```python
from build123d import *

# Parameters (mm, degrees)
SKETCH1_W                       = 243.332
SKETCH1_H                       = 49.394999
BOSS_EXTRUDE1_DEPTH             = 1.905
SKETCH2_W                       = 8.466666667
SKETCH2_H                       = 8.466666667
SKETCH2_W_2                     = 8.466666666
BOSS_EXTRUDE2_DEPTH             = 9.525
CUT_EXTRUDE1_DEPTH              = 6.35
CHAMFER1_SIZE                   = 0.635
BOSS_EXTRUDE3_START             = -234.865333
BOSS_EXTRUDE3_DEPTH             = 234.865333
F_6_CLEARANCE_HOLE1_D           = 4.3053
F_6_CLEARANCE_HOLE1_CSINK_D     = 6.35
F_6_CLEARANCE_HOLE1_CSINK_ANGLE = 90


with BuildPart() as part:
    # Sketch1 → Boss-Extrude1 (new body)
    with BuildSketch(Plane.XY):
        with Locations((121.666, 24.6974995)):
            Rectangle(SKETCH1_W, SKETCH1_H)
    extrude(amount=BOSS_EXTRUDE1_DEPTH)

    # Sketch2 → Boss-Extrude2 (add)
    with BuildSketch(Plane.XY):
        with Locations((4.233333334, 45.161665666)):
            Rectangle(SKETCH2_W, SKETCH2_H)
        with Locations((127, 45.161665666)):
            Rectangle(SKETCH2_W_2, SKETCH2_H)
        with Locations((213.698666667, 45.161665666)):
            Rectangle(SKETCH2_W, SKETCH2_H)
    extrude(amount=-BOSS_EXTRUDE2_DEPTH)

    # Sketch3 → Cut-Extrude1 (cut)
    with BuildSketch(Plane(origin=(0, 49.394999, 0), x_dir=(1, 0, 0), z_dir=(0, 1, 0))):
        Polygon((1.058333333, 5.291666667), (4.233333333, 8.466666667), (7.408333333, 5.291666667), (4.233333333, 2.116666667), align=None)
        Polygon((123.825, 5.291666667), (127, 8.466666667), (130.175, 5.291666667), (127, 2.116666667), align=None)
        Polygon((210.523666667, 5.291666667), (213.698666667, 8.466666667), (216.873666667, 5.291666667), (213.698666667, 2.116666667), align=None)
    extrude(amount=-CUT_EXTRUDE1_DEPTH, mode=Mode.SUBTRACT)

    # Chamfer1
    chamfer1_edges = [part.edges().sort_by_distance(p)[0] for p in [
        (2.645833333, 43.044999, -3.704166667),
        (2.645833333, 43.044999, -6.879166667),
        (5.820833333, 43.044999, -6.879166667),
        (5.820833333, 43.044999, -3.704166667),
        (2.645833333, 49.394999, -3.704166667),
        (5.820833333, 49.394999, -3.704166667),
        (5.820833333, 49.394999, -6.879166667),
        (2.645833333, 49.394999, -6.879166667),
        (125.4125, 43.044999, -3.704166667),
        (125.4125, 43.044999, -6.879166667),
        (128.5875, 43.044999, -6.879166667),
        (128.5875, 43.044999, -3.704166667),
        (125.4125, 49.394999, -3.704166667),
        (128.5875, 49.394999, -3.704166667),
        (128.5875, 49.394999, -6.879166667),
        (125.4125, 49.394999, -6.879166667),
        (212.111166667, 43.044999, -3.704166667),
        (212.111166667, 43.044999, -6.879166667),
        (215.286166667, 43.044999, -6.879166667),
        (215.286166667, 43.044999, -3.704166667),
        (212.111166667, 49.394999, -3.704166667),
        (215.286166667, 49.394999, -3.704166667),
        (215.286166667, 49.394999, -6.879166667),
        (212.111166667, 49.394999, -6.879166667),
    ]]
    chamfer(chamfer1_edges, length=CHAMFER1_SIZE)


with BuildPart() as boss_extrude3_tool:
    # Sketch4 → Boss-Extrude3 (new body)
    with BuildSketch(Plane(origin=(243.332, 0, 0), x_dir=(0, 0, -1), z_dir=(1, 0, 0)).offset(BOSS_EXTRUDE3_START)):
        Polygon((0, 49.394999), (0.635, 49.394999), (0, 48.759999), align=None)
    extrude(amount=BOSS_EXTRUDE3_DEPTH)


with BuildPart() as part_1:
    add(part.part)


with BuildPart() as part_2:
    # Boss-Extrude3: joined with boss_extrude3_tool
    add(part_1.part.fuse(boss_extrude3_tool.part, tol=0.00001))

    # #6 Clearance Hole1 (through all)
    with Locations(Plane.XY.offset(1.905)):
        with Locations((9.525, 9.525), (233.807, 9.525)):
            CounterSinkHole(F_6_CLEARANCE_HOLE1_D / 2, F_6_CLEARANCE_HOLE1_CSINK_D / 2, counter_sink_angle=F_6_CLEARANCE_HOLE1_CSINK_ANGLE)


solid = part_2.part
```
Build history of the part. All positions in model axes, mm. A direction names the side the tool comes from. Give positions to 0.01 mm unless a question says otherwise; leave off trailing zeros. Loops run counter-clockwise (first coordinate to the right, second up) from the corner with the lowest first, then second, coordinate; pieces in that order, holes last. Notation, with made-up numbers: (21.25, -26) - (29.25, -26) arc R10 ccw to (29.25, -19) - close; hole circle Ø9 at (17, 78). An arc over 180 degrees is marked (long way). Use a Markdown table: item, result.
(1) Pull direction Z, two halves, no side cores. Call faces 4 (the face through (214, 40.928, -5)), 5 (the face through (4, 45, -9.525)), 6 (the face through (2.4, 49.07, -7.07)): +Z half, -Z half, draft (parallel to the pull), parting line (faces both ways), or undercut.
Taken from the geometry:
| item | result |
|---|---|
| face 4 | draft |
| face 5 | -Z half |
| face 6 | undercut |
(2) Band-saw the part on C-C (y = 22). Give the cut face in (x, z) (3 decimals).
Taken from the geometry:
| item | result |
|---|---|
| outline | (0, 0) - (243.332, 0) - (243.332, 1.905) - (0, 1.905) - close |
(3) Band-saw the part on B-B (x = 97.5). Give the cut face in (y, z) (3 decimals).
Taken from the geometry:
| item | result |
|---|---|
| outline | (0, 0) - (48.76, 0) - (49.395, -0.635) - (49.395, 1.905) - (0, 1.905) - close |
(4) Drop flat-ended pins along their axis: pin 1 Ø4 at (y, z) = (43, -3.5) entering from +X; pin 2 Ø2.5 at (x, z) = (126, -5) entering from +Y; pin 3 Ø5 at (x, y) = (9.525, 9.525) entering from +Z; pin 4 Ø5 at (x, z) = (5, -6.5) entering from +Y (3 decimals). Give the stop position or say it passes through.
Taken from the geometry:
| item | result |
|---|---|
| pin 1 | x = 217.93 |
| pin 2 | y = 43.6 |
| pin 3 | z = 1.23 |
| pin 4 | y = 49.395 |
(5) Band-saw the part on A-A (y = 46). Give the cut face in (x, z) (3 decimals), and give its area (3 significant figures).
Taken from the geometry:
| item | result |
|---|---|
| outline | (0, -9.525) - (8.467, -9.525) - (8.467, 0) - (122.767, 0) - (122.767, -9.525) - (131.233, -9.525) - (131.233, 0) - (209.465, 0) - (209.465, -9.525) - (217.932, -9.525) - (217.932, 0) - (243.332, 0) - (243.332, 1.905) - (0, 1.905) - close; hole (1.058, -5.292) - (4.233, -8.467) - (7.408, -5.292) - (4.233, -2.117) - close; hole (123.825, -5.292) - (127, -8.467) - (130.175, -5.292) - (127, -2.117) - close; hole (210.524, -5.292) - (213.699, -8.467) - (216.874, -5.292) - (213.699, -2.117) - close |
| area | 645 mm2 |
(6) Wall check: line 1 along Z through (x, y) = (80, 19.5) (3 decimals); line 2 along X through (y, z) = (46.5, -8.25); line 3 along X through (y, z) = (8, 0.5). Give the ranges that are in metal, low to high.
Taken from the geometry:
| item | result |
|---|---|
| line 1 | 0 to 1.905 |
| line 2 | 0 to 4.02, 4.45 to 8.47, 122.77 to 126.78, 127.22 to 131.23, 209.47 to 213.48, 213.92 to 217.93 |
| line 3 | 0 to 8.01, 11.04 to 232.29, 235.33 to 243.33 |
(7) Which spindle directions (+Z, -Z, +X, -X, +Y, -Y) get a long thin tool onto all of the face, cutting with end or side? Do faces 1 (the face through (130, 49.395, 0)), 2 (the face through (4, 40.928, -5)), 3 (the face through (215.536, 49.073, -3.511)). Say none if no direction does.
Taken from the geometry:
| item | result |
|---|---|
| face 1 | +Z, -Z, +X, -X, +Y |
| face 2 | -Z, +X, -X, -Y |
| face 3 | +Y |
